```python
from build123d import *

# Parameters (mm, degrees)
SKETCH1_W           = 70
SKETCH1_H           = 119
BOSS_EXTRUDE1_DEPTH = 35
SKETCH2_R           = 8
CUT_EXTRUDE1_DEPTH  = 8
SKETCH3_R           = 8
CUT_EXTRUDE2_DEPTH  = 8
SKETCH4_W           = 14
SKETCH4_H           = 89
CUT_EXTRUDE3_DEPTH  = 32
CUT_EXTRUDE4_REACH  = 82.804
CUT_EXTRUDE5_REACH  = 82.804
SKETCH7_W           = 23
SKETCH7_H           = 20
SKETCH7_W_2         = 16
CUT_EXTRUDE6_DEPTH  = 78.396705356
CUT_EXTRUDE7_DEPTH  = 5
SKETCH9_W           = 18
SKETCH9_H           = 32
CUT_EXTRUDE8_DEPTH  = 2
SKETCH10_W          = 24
SKETCH10_H          = 32
CUT_EXTRUDE9_DEPTH  = 2
SKETCH11_W          = 23
SKETCH11_H          = 32
CUT_EXTRUDE10_DEPTH = 2
SKETCH12_W          = 32
SKETCH12_H          = 20
CUT_EXTRUDE11_DEPTH = 2
SKETCH13_W          = 32
SKETCH13_H          = 20
CUT_EXTRUDE12_DEPTH = 2
SKETCH14_W          = 65
SKETCH14_H          = 32
CUT_EXTRUDE13_DEPTH = 2
SKETCH15_W          = 16
SKETCH15_H          = 32
CUT_EXTRUDE15_DEPTH = 2
SKETCH17_W          = 32
SKETCH17_H          = 20
CUT_EXTRUDE16_DEPTH = 2
SKETCH18_W          = 32
SKETCH18_H          = 20
CUT_EXTRUDE17_DEPTH = 2
SKETCH20_W          = 32
SKETCH20_H          = 95
CUT_EXTRUDE18_DEPTH = 5
SKETCH21_R          = 1.5
CUT_EXTRUDE20_DEPTH = 10
FILLET1_R           = 5
FILLET2_R           = 5


with BuildPart() as part:
    # Sketch1 → Boss-Extrude1 (new body)
    with BuildSketch(Plane.XY):
        Rectangle(SKETCH1_W, SKETCH1_H)
    extrude(amount=BOSS_EXTRUDE1_DEPTH)

    # Sketch2 → Cut-Extrude1 (cut)
    with BuildSketch(Plane(origin=(35, 0, 0), x_dir=(0, 0, -1), z_dir=(1, 0, 0))):
        with Locations((0, -19.5)):
            Circle(SKETCH2_R)
    extrude(amount=-CUT_EXTRUDE1_DEPTH, mode=Mode.SUBTRACT)

    # Sketch3 → Cut-Extrude2 (cut)
    with BuildSketch(Plane.ZY.offset(35)):
        with Locations((0, 19.5)):
            Circle(SKETCH3_R)
    extrude(amount=-CUT_EXTRUDE2_DEPTH, mode=Mode.SUBTRACT)

    # Sketch4 → Cut-Extrude3 (cut)
    with BuildSketch(Plane(origin=(0, 0, 0), x_dir=(-1, 0, 0), z_dir=(0, 0, -1))):
        with Locations((-20, 9.526034086)):
            Rectangle(SKETCH4_W, SKETCH4_H)
        with Locations((0, -10)):
            Rectangle(SKETCH4_W, SKETCH4_H)
        with Locations((20, 9.526034086)):
            Rectangle(SKETCH4_W, SKETCH4_H)
    extrude(amount=-CUT_EXTRUDE3_DEPTH, mode=Mode.SUBTRACT)

    # Sketch5 → Cut-Extrude4 (cut, up to next)
    with BuildSketch(Plane.ZY.offset(-7), mode=Mode.PRIVATE) as cut_extrude4_sk1:
        with BuildLine():
            Line((0, 27.5), (0, 11.5))
            ThreePointArc((0, 11.5), (8, 19.5), (0, 27.5))
        make_face()
    cut_extrude4_tool1 = extrude(cut_extrude4_sk1.sketch, amount=-CUT_EXTRUDE4_REACH, mode=Mode.PRIVATE) & part.part
    add(cut_extrude4_tool1.solids().sort_by_distance((7, 19.5, 3.395305))[0], mode=Mode.SUBTRACT)

    # Sketch6 → Cut-Extrude5 (cut, up to next)
    with BuildSketch(Plane(origin=(-7, 0, 0), x_dir=(0, 0, -1), z_dir=(1, 0, 0)), mode=Mode.PRIVATE) as cut_extrude5_sk1:
        with BuildLine():
            Line((0, -27.5), (0, -11.5))
            ThreePointArc((0, -11.5), (-8, -19.5), (0, -27.5))
        make_face()
    cut_extrude5_tool1 = extrude(cut_extrude5_sk1.sketch, amount=-CUT_EXTRUDE5_REACH, mode=Mode.PRIVATE) & part.part
    add(cut_extrude5_tool1.solids().sort_by_distance((-7, -19.5, 3.395305))[0], mode=Mode.SUBTRACT)

    # Sketch7 → Cut-Extrude6 (cut, through all)
    with BuildSketch(Plane(origin=(0, 0, 0), x_dir=(-1, 0, 0), z_dir=(0, 0, -1))):
        with Locations((23.5, -49.5)):
            Rectangle(SKETCH7_W, SKETCH7_H)
        with Locations((0, 49.5)):
            Rectangle(SKETCH7_W_2, SKETCH7_H)
        with Locations((-23.5, -49.5)):
            Rectangle(SKETCH7_W, SKETCH7_H)
    extrude(amount=-CUT_EXTRUDE6_DEPTH, mode=Mode.SUBTRACT)

    # Sketch8 → Cut-Extrude7 (cut)
    with BuildSketch(Plane(origin=(35, 0, 0), x_dir=(0, 0, -1), z_dir=(1, 0, 0))):
        with BuildLine():
            Line((-3, 59.5), (-35, 59.5))
            Line((-35, 59.5), (-35, -39.5))
            Line((-35, -39.5), (-3, -39.5))
            Line((-3, -39.5), (-3, -30.083005244))
            ThreePointArc((-3, -30.083005244), (-11, -19.5), (-3, -8.916994756))
            Line((-3, -8.916994756), (-3, 59.5))
        make_face()
    extrude(amount=-CUT_EXTRUDE7_DEPTH, mode=Mode.SUBTRACT)

    # Sketch9 → Cut-Extrude8 (cut)
    with BuildSketch(Plane.XZ.offset(39.5)):
        with Locations((21, 19)):
            Rectangle(SKETCH9_W, SKETCH9_H)
    extrude(amount=-CUT_EXTRUDE8_DEPTH, mode=Mode.SUBTRACT)

    # Sketch10 → Cut-Extrude9 (cut)
    with BuildSketch(Plane.XZ.offset(59.5)):
        with Locations((0, 19)):
            Rectangle(SKETCH10_W, SKETCH10_H)
    extrude(amount=-CUT_EXTRUDE9_DEPTH, mode=Mode.SUBTRACT)

    # Sketch11 → Cut-Extrude10 (cut)
    with BuildSketch(Plane.XZ.offset(39.5)):
        with Locations((-23.5, 19)):
            Rectangle(SKETCH11_W, SKETCH11_H)
    extrude(amount=-CUT_EXTRUDE10_DEPTH, mode=Mode.SUBTRACT)

    # Sketch12 → Cut-Extrude11 (cut)
    with BuildSketch(Plane.ZY.offset(12)):
        with Locations((19, -47.5)):
            Rectangle(SKETCH12_W, SKETCH12_H)
    extrude(amount=-CUT_EXTRUDE11_DEPTH, mode=Mode.SUBTRACT)

    # Sketch13 → Cut-Extrude12 (cut)
    with BuildSketch(Plane(origin=(12, 0, 0), x_dir=(0, 0, -1), z_dir=(1, 0, 0))):
        with Locations((-19, -47.5)):
            Rectangle(SKETCH13_W, SKETCH13_H)
    extrude(amount=-CUT_EXTRUDE12_DEPTH, mode=Mode.SUBTRACT)

    # Sketch14 → Cut-Extrude13 (cut)
    with BuildSketch(Plane(origin=(0, 59.5, 0), x_dir=(1, 0, 0), z_dir=(0, 1, 0))):
        with Locations((-2.5, -19)):
            Rectangle(SKETCH14_W, SKETCH14_H)
    extrude(amount=-CUT_EXTRUDE13_DEPTH, mode=Mode.SUBTRACT)

    # Sketch15 → Cut-Extrude15 (cut)
    with BuildSketch(Plane(origin=(0, 39.5, 0), x_dir=(1, 0, 0), z_dir=(0, 1, 0))):
        with Locations((0, -19)):
            Rectangle(SKETCH15_W, SKETCH15_H)
    extrude(amount=-CUT_EXTRUDE15_DEPTH, mode=Mode.SUBTRACT)

    # Sketch17 → Cut-Extrude16 (cut)
    with BuildSketch(Plane(origin=(-8, 0, 0), x_dir=(0, 0, -1), z_dir=(1, 0, 0))):
        with Locations((-19, 47.5)):
            Rectangle(SKETCH17_W, SKETCH17_H)
    extrude(amount=-CUT_EXTRUDE16_DEPTH, mode=Mode.SUBTRACT)

    # Sketch18 → Cut-Extrude17 (cut)
    with BuildSketch(Plane.ZY.offset(-8)):
        with Locations((19, 47.5)):
            Rectangle(SKETCH18_W, SKETCH18_H)
    extrude(amount=-CUT_EXTRUDE17_DEPTH, mode=Mode.SUBTRACT)

    # Sketch20 → Cut-Extrude18 (cut)
    with BuildSketch(Plane.ZY.offset(35)):
        with Locations((19, 10)):
            Rectangle(SKETCH20_W, SKETCH20_H)
    extrude(amount=-CUT_EXTRUDE18_DEPTH, mode=Mode.SUBTRACT)

    # Sketch21 → Cut-Extrude20 (cut)
    with BuildSketch(Plane(origin=(0, 0, 0), x_dir=(-1, 0, 0), z_dir=(0, 0, -1))):
        with Locations((-32, 56.5)):
            Circle(SKETCH21_R)
        with Locations((32, 56.5)):
            Circle(SKETCH21_R)
        with Locations((32, -36.5)):
            Circle(SKETCH21_R)
        with Locations((-32, -36.5)):
            Circle(SKETCH21_R)
    extrude(amount=-CUT_EXTRUDE20_DEPTH, mode=Mode.SUBTRACT)

    # Fillet1
    fillet1_edges = [part.edges().sort_by_distance(p)[0] for p in [
        (30, -37.5, 19),
        (-10, -57.5, 19),
        (-10, -37.5, 19),
        (10, -37.5, 19),
        (10, -57.5, 19),
        (30, 57.5, 19),
        (-10, 37.5, 19),
        (-10, 57.5, 19),
        (10, 57.5, 19),
        (10, 37.5, 19),
        (-30, 57.5, 19),
        (-30, -37.5, 19),
    ]]
    fillet(fillet1_edges, radius=FILLET1_R)

    # Fillet2
    fillet2_edges = [part.edges().sort_by_distance(p)[0] for p in [
        (35, 59.5, 1.5),
        (8, 59.5, 1.5),
        (-8, 59.5, 1.5),
        (-35, 59.5, 1.5),
        (-35, 11.64730658, 1.5281381),
        (-35, 27.35269342, 1.5281381),
        (-35, -39.5, 1.5),
        (-12, -59.5, 1.5),
        (12, -59.5, 1.5),
        (35, -39.5, 1.5),
    ]]
    fillet(fillet2_edges, radius=FILLET2_R)


solid = part.part
```
Model file for the job. Use its own axes, mm. A direction names the side the tool comes from. Coordinates: 2 decimals unless noted, no trailing zeros. Loops run counter-clockwise (first coordinate to the right, second up) from the corner with the lowest first, then second, coordinate; pieces in that order, holes last. Notation, with made-up numbers: (82.25, 80) -> (95.25, 80) arc R14 ccw to (95.25, 85) -> close; hole circle Ø8 at (87.25, 63). An arc over 180 degrees is marked (long way). Answer as a JSON object with one key per item and string values.
Q1. Cut at A-A (y = -19.5). List the corners of the cut face in (x, z).
Report:
{"outline": "(-35, 0) -> (-27, 0) -> (-27, 32) -> (-13, 32) -> (-13, 8) -> (-7, 8) -> (-7, 32) -> (7, 32) -> (7, 0) -> (13, 0) -> (13, 32) -> (27, 32) -> (27, 8) -> (35, 8) -> (35, 11) -> (30, 11) -> (30, 35) -> (-30, 35) -> (-30, 3) -> (-35, 3) -> close"}
Q2. Cut at C-C (z = 19). State how many separate pieces and enclosed holes the cut face has, and give its area (3 significant figures).
Report:
{"separate pieces": "1", "enclosed holes": "3", "area": "1,940 mm2"}
Q3. Cut at D-D (y = 36). List the corners of the cut face in (x, z).
Report:
{"outline": "(-35, 0) -> (-27, 0) -> (-27, 32) -> (-13, 32) -> (-13, 0) -> (13, 0) -> (13, 32) -> (27, 32) -> (27, 0) -> (35, 0) -> (35, 3) -> (30, 3) -> (30, 35) -> (-30, 35) -> (-30, 3) -> (-35, 3) -> close"}
Q4. Flat gauge pins, fed straight in: P1, Ø4, axis at x = 2.5, z = 22.5, coming from the -Y side; P2, Ø5, axis at x = -32, y = 56.5, coming from the +Z side; P3, Ø4, axis at x = 0.5, y = 30, coming from the -Z side; P4, Ø1.5, axis at x = 13.5, y = 42, coming from the -Z side. Where does each tip first touch, or does it go through?
Report:
{"P1": "stops at y = -57.5", "P2": "stops at z = 3", "P3": "stops at z = 32", "P4": "stops at z = 0"}
Q5. 3-axis set-ups, long thin cutter, end or side, ignore diameter. For faces 4 (the flat face through (10, 48, 19)), 5 (the flat face through (-27, 9, 16)), 6 (the flat face through (8, 47, 1)): which of +Z, -Z, +X, -X, +Y, -Y reach the whole face in a straight line?
Report:
{"face 4": "+Z, +Y", "face 5": "-Z", "face 6": "+Z, -Z, +Y"}
Q6. Probe probe 1 along X at (y, z) = (11.5, 21.5); probe 2 along X at (y, z) = (36, 30); probe 3 along X at (y, z) = (42.5, 4). List the from-to ranges inside material, lowest first.
Report:
{"probe 1": "x = -30 to -27, -13 to -7, 7 to 13, 27 to 30", "probe 2": "x = -30 to -27, -13 to 13, 27 to 30", "probe 3": "x = -30 to -27, -13 to -10, 10 to 13, 27 to 30"}
Q7. Cut at B-B (x = 23). List the corners of the cut face in (y, z).
Report:
{"outline": "(-39.5, 0) -> (-34.97, 0) -> (-34.97, 32) -> (54.03, 32) -> (54.03, 0) -> (59.5, 0) -> (59.5, 3) -> (57.5, 3) -> (57.5, 35) -> (-37.5, 35) -> (-37.5, 3) -> (-39.5, 3) -> close"}
Q8. Pull direction X, two halves, no side cores. Call faces 1 (the cylindrical face through (-8.57, -56, 19.22)), 2 (the cylindrical face through (10.5, -58.07, 1.52)), 3 (the cylindrical face through (-9.5, 58.07, 1.52)): released by +X, released by -X, zero draft, split by the parting line, or undercut.
Report:
{"face 1": "released by -X", "face 2": "released by +X", "face 3": "undercut"}
